```python
from build123d import *

# Parameters (mm, degrees)
SKETCH1_W           = 579
SKETCH1_H           = 459
BOSS_EXTRUDE1_DEPTH = 2.2479
CUT_EXTRUDE1_DEPTH  = 4.4958


with BuildPart() as part:
    # Sketch1 → Boss-Extrude1 (new body, symmetric)
    with BuildSketch(Plane.XY):
        Rectangle(SKETCH1_W, SKETCH1_H)
    extrude(amount=BOSS_EXTRUDE1_DEPTH, both=True)

    # Sketch2 → Cut-Extrude1 (cut)
    with BuildSketch(Plane(origin=(0, 0, -2.2479), x_dir=(-1, 0, 0), z_dir=(0, 0, -1))):
        Polygon((-280.249993563, -59.7), (-290, -59.7), (-290, -230), (-59.249993563, -230), (-59.249993563, -221.7), (-62.249993563, -221.7), (-62.249993563, -102.7), (-59.249993563, -102.7), (-59.249993563, -99.7), (-236.249993563, -99.7), (-236.249993563, -95.7), (-280.249993563, -95.7), align=None)
    extrude(amount=-CUT_EXTRUDE1_DEPTH, mode=Mode.SUBTRACT)


solid = part.part
```
Geometry check sheet. Reference: the model listing, model coordinates, mm. Round coordinates to 2 decimals unless told otherwise and drop trailing zeros. Loops run counter-clockwise (first coordinate to the right, second up) from the corner with the lowest first, then second, coordinate; pieces in that order, holes last. Notation, with made-up numbers: (51.5, -23) - (95.5, -23) arc R31 cw to (95.5, 7) - close; hole circle Ø6 at (54.25, 52). An arc over 180 degrees is marked (long way). Write each question's results on one line, items separated by ' | '. Start each with the question number.
Q1. Gauge pin test, flat ends, axial feed: P1, Ø2, axis at y = -168.5, z = -1, coming from the +X side; P2, Ø0.9, axis at x = 61, z = 1, coming from the -Y side; P3, Ø1.3, axis at y = -227, z = -0.5, coming from the +X side. Record the tip position at first contact, or that the pin passes through.
Q2. Cross-section at B-B on y = -111.5. Enter the section's corners in (x, z), and give its area (3 significant figures).
Q3. Cross-section at A-A on z = 0.55. Enter the section's corners in (x, y), and give its area (3 significant figures).
Q4. Thickness scan on line 1 (X direction, y = -143.5, z = -1.6); line 2 (Y direction, x = 156.5, z = 0.05). Record the ranges inside material, lowest first. Write a range as [from, to].
Q5. Cross-section at C-C on x = 84.5. Enter the section's corners in (y, z), and give its area (3 significant figures).
Answers below:
1) P1: stops at x = 62.25 | P2: stops at y = -221.7 | P3: stops at x = 59.25
2) outline: (-289.5, -2.25) - (62.25, -2.25) - (62.25, 2.25) - (-289.5, 2.25) - close | area: 1,580 mm²
3) outline: (-289.5, -229.5) - (59.25, -229.5) - (59.25, -221.7) - (62.25, -221.7) - (62.25, -102.7) - (59.25, -102.7) - (59.25, -99.7) - (236.25, -99.7) - (236.25, -95.7) - (280.25, -95.7) - (280.25, -59.7) - (289.5, -59.7) - (289.5, 229.5) - (-289.5, 229.5) - close | area: 236,000 mm²
4) line 1: x = [-289.5, 62.25] | line 2: y = [-99.7, 229.5]
5) outline: (-99.7, -2.25) - (229.5, -2.25) - (229.5, 2.25) - (-99.7, 2.25) - close | area: 1,480 mm²
